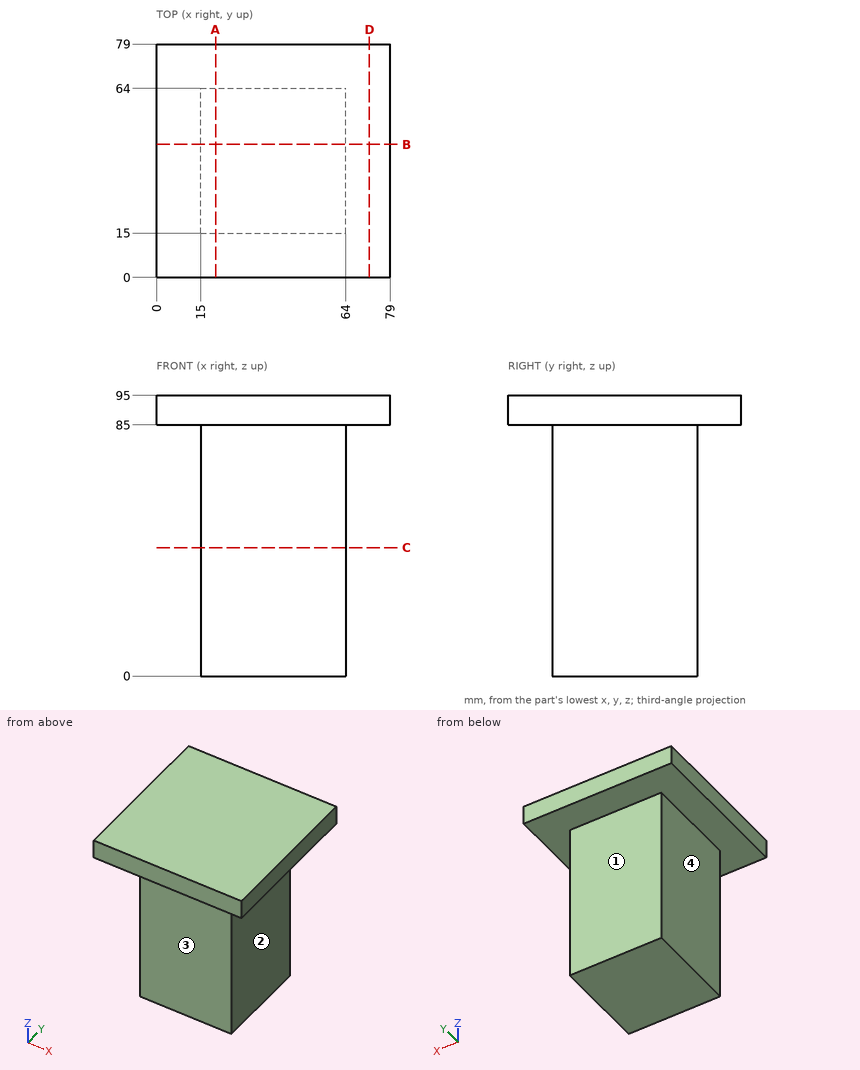
The figure shows three views and two pictorial views of one solid part (mm, origin at its lowest corner). Answer the questions. A direction names the side the tool comes from. Coordinates: 2 decimals unless noted, no trailing zeros. Loops run counter-clockwise (first coordinate to the right, second up) from the corner with the lowest first, then second, coordinate; pieces in that order, holes last. Notation, with made-up numbers: (35, -24.5) -> (47, -24.5) arc R22 cw to (47, -0.5) -> close; hole circle Ø4 at (25.5, -19). An arc over 180 degrees is marked (long way). Write item = value, one per line. Start each with the question number.
1) A cutting plane is placed at C-C (z = 43.5). Give the vertices of the cut face in (x, y).
2) Given pin 1 Ø24.5 at (y, z) = (38.5, 27.5) entering from -X; pin 2 Ø1 at (x, z) = (54.5, 10.5) entering from -Y; pin 3 Ø10 at (x, z) = (56, 11.5) entering from +Y, each flat-ended and moving along its own axis, determine where each tip first touches the part or whether it passes through.
3) Straight lines are drawn through the part: line 1 (Y direction, x = 35, z = 71); line 2 (Z direction, x = 54.5, y = 75). For each, find the intervals that lie inside material, in ascending order. Write a range as from..to.
4) A tool of negligible diameter and unlimited length cuts with its end or side. For the marked faces 1, 2, 3 and 4, from which of +Z, -Z, +X, -X, +Y, -Y can it reach the whole face along a straight path? Write none if from no direction.
5) A cutting plane is placed at A-A (x = 20). Give the vertices of the cut face in (y, z), then the cut area to 4 significant figures.
6) A cutting plane is placed at D-D (x = 72). Give the vertices of the cut face in (y, z).
Responses:
q1.outline = (15, 15) -> (64, 15) -> (64, 64) -> (15, 64) -> close
q2.pin_1 = 15
q2.pin_2 = 15
q2.pin_3 = 64
q3.line_1 = 15..64
q3.line_2 = 85..95
q4.face_1 = -Z, +X, -X, +Y
q4.face_2 = -Z, +X, +Y, -Y
q4.face_3 = -Z, +X, -X, -Y
q4.face_4 = -Z, -X, +Y, -Y
q5.outline = (0, 85) -> (15, 85) -> (15, 0) -> (64, 0) -> (64, 85) -> (79, 85) -> (79, 95) -> (0, 95) -> close
q5.area = 4,955 mm²
q6.outline = (0, 85) -> (79, 85) -> (79, 95) -> (0, 95) -> close
